Work out the finished part from the listing and answer in its coordinate system (mm). A direction names the side the tool comes from. Coordinates: 2 decimals unless noted, no trailing zeros. Order: outer loops, then holes, each group sorted by start corner. A loop starts at its lowest first (then second) coordinate and runs counter-clockwise, first axis right, second up.
1. The part is cut by section D-D, the plane y = -23.5. Give the vertices of the cut face in (x, z).
2. The part is cut by section C-C, the plane x = -32.5. Give the vertices of the cut face in (y, z), then the cut area to 3 significant figures.
3. Find the intervals of material crossed by probe 1 along Z at (x, y) = (-32.5, -11.25); probe 2 along X at (y, z) = (-9, 9.75); probe 3 along X at (y, z) = (-12, 4), in increasing order.
4. A tool of negligible diameter and unlimited length cuts with its end or side. For faces 1 (the flat face through (38, -20, 7)), 2 (the flat face through (-38, -20, 7)), 3 (the flat face through (1, -29, 0)), from which of +Z, -Z, +X, -X, +Y, -Y can it reach the whole face along a straight path? Write none if from no direction.
5. The part is cut by section A-A, the plane z = 7.5. Give the vertices of the cut face in (x, y), then the cut area to 3 significant figures.
6. Flat-ended cylindrical pins translate along their axes: pin 1 Ø1 at (x, z) = (-9.5, 7) entering from -Y; pin 2 Ø1 at (x, y) = (7.5, -26.5) entering from -Z; pin 3 Ø6 at (x, z) = (32.5, 7.5) entering from +Y; pin 4 Ø1.5 at (y, z) = (-24, 9.5) entering from +X. Find the tip coordinate at first contact, or state that the pin passes through.
7. The part is cut by section B-B, the plane y = -15.5. Give the vertices of the cut face in (x, z), then the cut area to 3 significant figures.
8. Determine the mould class of faces 4 (the cylindrical face through (27.505, -11.093, 7.28)), 5 (the cylindrical face through (-27.881, -11.093, 9.415)), 6 (the flat face through (40, -10, 7)), 7 (the flat face through (1, -29, 15)) for opening direction X: +X half, -X half, draft (parallel to the pull), parting line (faces both ways), or undercut.
```python
from build123d import *

# Parameters (mm, degrees)
BOSS_EXTRUDE4_DEPTH = 15
SKETCH5_R           = 5
CUT_EXTRUDE1_DEPTH  = 41


with BuildPart() as part:
    # Sketch2 → Boss-Extrude4 (new body)
    with BuildSketch(Plane.XY):
        with BuildLine():
            Line((-40, 0), (-25, 0))
            ThreePointArc((-25, 0), (0, -25), (25, 0))
            Line((25, 0), (40, 0))
            Line((40, 0), (40, -20))
            Line((40, -20), (34.641016151, -20))
            ThreePointArc((34.641016151, -20), (0, -40), (-34.641016151, -20))
            Line((-34.641016151, -20), (-40, -20))
            Line((-40, -20), (-40, 0))
        make_face()
    extrude(amount=BOSS_EXTRUDE4_DEPTH)

    # Sketch5 → Cut-Extrude1 (cut, through all)
    with BuildSketch(Plane(origin=(0, 0, 0), x_dir=(1, 0, 0), z_dir=(0, 1, 0))):
        with Locations((-32.5, -7.5)):
            Circle(SKETCH5_R)
        with Locations((32.5, -7.5)):
            Circle(SKETCH5_R)
    extrude(amount=-CUT_EXTRUDE1_DEPTH, mode=Mode.SUBTRACT)


solid = part.part
```
Geometry says:
1. outline: (-32.37, 0) - (-8.53, 0) - (-8.53, 15) - (-32.37, 15) - (-32.37, 12.5) arc R5 cw to (-32.37, 2.5) - close; (8.53, 0) - (32.37, 0) - (32.37, 2.5) arc R5 cw to (32.37, 12.5) - (32.37, 15) - (8.53, 15) - close
2. outline: (-23.32, 0) - (0, 0) - (0, 2.5) - (-23.32, 2.5) - close; (-23.32, 12.5) - (0, 12.5) - (0, 15) - (-23.32, 15) - close
2. area: 117 mm2
3. probe 1: z = 0 to 2.5, 12.5 to 15
3. probe 2: x = -40 to -36.97, -28.03 to -23.32, 23.32 to 28.03, 36.97 to 40
3. probe 3: x = -40 to -36.07, -28.93 to -21.93, 21.93 to 28.93, 36.07 to 40
4. face 1: +Z, -Z, +X, -Y
4. face 2: +Z, -Z, -X, -Y
4. face 3: -Z, +X, -X, +Y, -Y
5. outline: (-40, -20) - (-37.5, -20) - (-37.5, 0) - (-40, 0) - close; (-27.5, -29.05) arc R40 ccw to (27.5, -29.05) - (27.5, 0) - (25, 0) arc R25 cw to (-25, 0) - (-27.5, 0) - close; (37.5, -20) - (40, -20) - (40, 0) - (37.5, 0) - close
5. area: 1,130 mm2
6. pin 1: stops at y = -38.97
6. pin 2: stops at z = 0
6. pin 3: passes through
6. pin 4: stops at x = 28.32
7. outline: (-40, 0) - (-19.62, 0) - (-19.62, 15) - (-40, 15) - close; (19.62, 0) - (40, 0) - (40, 15) - (19.62, 15) - close; hole circle Ø10 at (-32.5, 7.5); hole circle Ø10 at (32.5, 7.5)
7. area: 454 mm2
8. face 4: undercut
8. face 5: undercut
8. face 6: +X half
8. face 7: draft
